Drawing for the job (mm, zero at the part's lowest x, y, z). Coordinates: 2 decimals unless noted, no trailing zeros. Write each loop counter-clockwise with the first axis right and the second up, starting at its lowest first coordinate (ties: lowest second). Pieces come first, ordered by that corner, then holes.
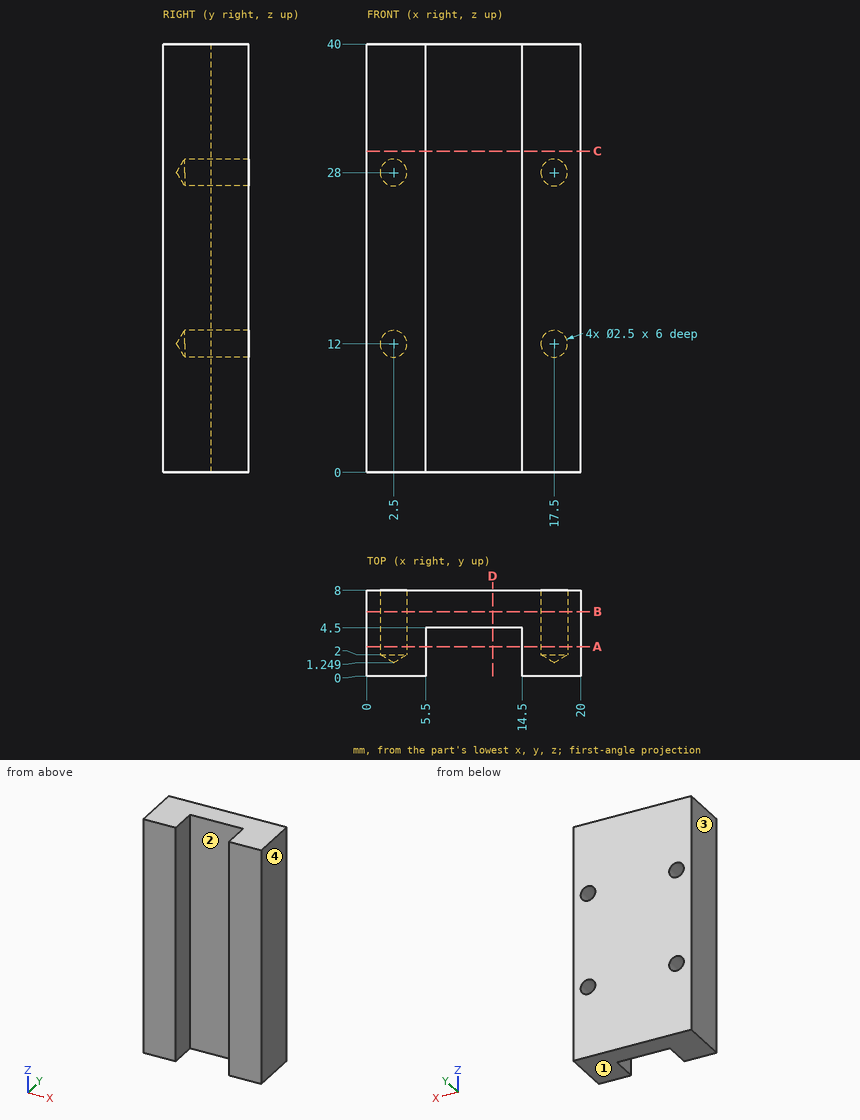
Item 1: Saw through at A-A, the plane y = 2.75. Write the cut outline in (x, z).
Item 2: Two-plate mould, pull along X, no slides. Class the marked faces 1, 2, 3 and 4: +X half, -X half, draft (parallel to the pull), parting line (faces both ways), or undercut.
Item 3: Saw through at D-D, the plane x = 11.75. Write the cut outline in (y, z).
Item 4: Saw through at C-C, the plane z = 30. Write the cut outline in (x, y).
Item 5: Wall check: line 1 along Z through (x, y) = (2.5, 4.15); line 2 along X through (y, z) = (5.6, 12); line 3 along X through (y, z) = (3.6, 12). Give the ranges that are in metal, low to high.
Item 6: Flat gauge pin, fed straight in: pin 1 Ø2.5 at (x, z) = (9, 13) entering from -Y. Where does the tip first touch, or does it go through?
Item 7: Saw through at B-B, the plane y = 6. Write the cut outline in (x, z).
Working result:
1. outline: (0, 0) - (5.5, 0) - (5.5, 40) - (0, 40) - close; (14.5, 0) - (20, 0) - (20, 40) - (14.5, 40) - close; hole circle Ø2.5 at (2.5, 12); hole circle Ø2.5 at (2.5, 28); hole circle Ø2.5 at (17.5, 12); hole circle Ø2.5 at (17.5, 28)
2. face 1: draft
2. face 2: undercut
2. face 3: -X half
2. face 4: +X half
3. outline: (4.5, 0) - (8, 0) - (8, 40) - (4.5, 40) - close
4. outline: (0, 0) - (5.5, 0) - (5.5, 4.5) - (14.5, 4.5) - (14.5, 0) - (20, 0) - (20, 8) - (0, 8) - close
5. line 1: z = 0 to 10.75, 13.25 to 26.75, 29.25 to 40
5. line 2: x = 0 to 1.25, 3.75 to 16.25, 18.75 to 20
5. line 3: x = 0 to 1.25, 3.75 to 5.5, 14.5 to 16.25, 18.75 to 20
6. pin 1: stops at y = 4.5
7. outline: (0, 0) - (20, 0) - (20, 40) - (0, 40) - close; hole circle Ø2.5 at (2.5, 12); hole circle Ø2.5 at (2.5, 28); hole circle Ø2.5 at (17.5, 12); hole circle Ø2.5 at (17.5, 28)
